Design review of the part built by this model. Coordinates are the model's own, in mm. A direction names the side the tool comes from. Round coordinates to 2 decimals unless told otherwise and drop trailing zeros. Loops run counter-clockwise (first coordinate to the right, second up) from the corner with the lowest first, then second, coordinate; pieces in that order, holes last. Notation, with made-up numbers: M 18,57 L 32,57 A29 ccw 32,96 Z; hole C -37.75,51 d7. An arc over 180 degrees is marked long. Use a Markdown table: item, result.
from build123d import *

# Parameters (mm, degrees)
SKETCH1_W           = 66.25
SKETCH1_H           = 78
SKETCH1_R           = 1.25
BOSS_EXTRUDE1_DEPTH = 3
SKETCH2_W           = 9.747388218
SKETCH2_H           = 78
SKETCH2_W_2         = 10.388237
BOSS_EXTRUDE2_DEPTH = 1.5
FILLET2_R           = 0.25
FILLET3_R           = 0.25
SKETCH3_R           = 2.3
SKETCH3_R_2         = 1.25
BOSS_EXTRUDE3_DEPTH = 4
SKETCH4_W           = 4.75
SKETCH4_H           = 3
BOSS_EXTRUDE4_DEPTH = 2
SKETCH5_W           = 5
SKETCH5_H           = 3
BOSS_EXTRUDE5_DEPTH = 30


with BuildPart() as part:
    # Sketch1 → Boss-Extrude1 (new body)
    with BuildSketch(Plane(origin=(0, 0, 0), x_dir=(1, 0, 0), z_dir=(0, 1, 0))):
        Rectangle(SKETCH1_W, SKETCH1_H)
        with Locations(Location((-21, 36, 0), (0, 0, 270))):
            Circle(SKETCH1_R, mode=Mode.SUBTRACT)
        with Locations(Location((21, 36, 0), (0, 0, 90))):
            Circle(SKETCH1_R, mode=Mode.SUBTRACT)
        with Locations(Location((21, -36, 0), (0, 0, 270))):
            Circle(SKETCH1_R, mode=Mode.SUBTRACT)
        with Locations(Location((-21, -36, 0), (0, 0, 90))):
            Circle(SKETCH1_R, mode=Mode.SUBTRACT)
    extrude(amount=BOSS_EXTRUDE1_DEPTH)

    # Sketch2 → Boss-Extrude2 (add)
    with BuildSketch(Plane.XZ):
        with Locations((-30.251305891, 0)):
            Rectangle(SKETCH2_W, SKETCH2_H)
        with Locations((29.9308815, 0)):
            Rectangle(SKETCH2_W_2, SKETCH2_H)
    extrude(amount=-BOSS_EXTRUDE2_DEPTH)

    # Fillet2
    fillet2_edges = [part.edges().sort_by_distance(p)[0] for p in [
        (-35.125, 0.75, 39),
        (-35.125, 0, 0),
        (-35.125, 1.5, 0),
        (-35.125, 0.75, -39),
    ]]
    fillet(fillet2_edges, radius=FILLET2_R)

    # Fillet3
    fillet3_edges = [part.edges().sort_by_distance(p)[0] for p in [
        (35.125, 0.75, -39),
        (35.125, 0, 0),
        (35.125, 1.5, 0),
        (35.125, 0.75, 39),
    ]]
    fillet(fillet3_edges, radius=FILLET3_R)

    # Sketch3 → Boss-Extrude3 (add)
    # profile 1 of 4: a face of its own
    with BuildSketch(Plane(origin=(0, 3, 0), x_dir=(1, 0, 0), z_dir=(0, 1, 0))):
        with Locations(Location((-21, 36, 0), (0, 0, 270))):
            Circle(SKETCH3_R)
        with Locations(Location((-21, 36, 0), (0, 0, 270))):
            Circle(SKETCH3_R_2, mode=Mode.SUBTRACT)
    # profile 2 of 4: a face of its own
    with BuildSketch(Plane(origin=(0, 3, 0), x_dir=(1, 0, 0), z_dir=(0, 1, 0))):
        with Locations(Location((21, 36, 0), (0, 0, 90))):
            Circle(SKETCH3_R)
        with Locations(Location((21, 36, 0), (0, 0, 90))):
            Circle(SKETCH3_R_2, mode=Mode.SUBTRACT)
    # profile 3 of 4: a face of its own
    with BuildSketch(Plane(origin=(0, 3, 0), x_dir=(1, 0, 0), z_dir=(0, 1, 0))):
        with Locations(Location((21, -36, 0), (0, 0, 270))):
            Circle(SKETCH3_R)
        with Locations(Location((21, -36, 0), (0, 0, 270))):
            Circle(SKETCH3_R_2, mode=Mode.SUBTRACT)
    # profile 4 of 4: a face of its own
    with BuildSketch(Plane(origin=(0, 3, 0), x_dir=(1, 0, 0), z_dir=(0, 1, 0))):
        with Locations(Location((-21, -36, 0), (0, 0, 90))):
            Circle(SKETCH3_R)
        with Locations(Location((-21, -36, 0), (0, 0, 90))):
            Circle(SKETCH3_R_2, mode=Mode.SUBTRACT)
    extrude(amount=BOSS_EXTRUDE3_DEPTH)

    # Sketch4 → Boss-Extrude4 (add)
    with BuildSketch(Plane.XY.offset(39)):
        with Locations((-20.925, 1.5)):
            Rectangle(SKETCH4_W, SKETCH4_H)
        with Locations((20.925, 1.5)):
            Rectangle(SKETCH4_W, SKETCH4_H)
    extrude(amount=BOSS_EXTRUDE4_DEPTH)

    # Sketch5 → Boss-Extrude5 (add)
    with BuildSketch(Plane(origin=(0, 0, -39), x_dir=(-1, 0, 0), z_dir=(0, 0, -1))):
        with Locations((-27.625, 1.5)):
            Rectangle(SKETCH5_W, SKETCH5_H)
        with Locations((27.625, 1.5)):
            Rectangle(SKETCH5_W, SKETCH5_H)
    extrude(amount=BOSS_EXTRUDE5_DEPTH)


solid = part.part
1. Machinability: for faces 4 (the face through (18.55, 1, 40)), 5 (the face through (30.125, 1, -54)), 6 (the face through (19.6, 4.972, 34.175)), 7 (the face through (-30.125, 1, -54)), which of the approach directions +Z, -Z, +X, -X, +Y, -Y give a long, thin tool a straight path to every point of the face, cutting with its end or side? Answer none if there is none.
Check values:
| item | result |
|---|---|
| face 4 | +Z, +Y, -Y |
| face 5 | -Z, +X, +Y, -Y |
| face 6 | +Y |
| face 7 | -Z, -X, +Y, -Y |
2. Wall thickness on line 1 along X through (y, z) = (6.75, -36); line 2 along X through (y, z) = (2, 36) (3 decimals); line 3 along X through (y, z) = (1.75, -62.5) (3 decimals): over which ranges is each line inside the solid? List them lowest first. Write a range as from..to.
Check values:
| item | result |
|---|---|
| line 1 | x = -23.3..-22.25, -19.75..-18.7, 18.7..19.75, 22.25..23.3 |
| line 2 | x = -33.125..-22.25, -19.75..19.75, 22.25..33.125 |
| line 3 | x = -30.125..-25.125, 25.125..30.125 |
3. Take a section at A-A on y = 5.75. Give the boundary of the cut face in (x, z).
Check values:
| item | result |
|---|---|
| outline | C -21,-36 d4.6; C -21,36 d4.6; C 21,-36 d4.6; C 21,36 d4.6; hole C -21,-36 d2.5; hole C -21,36 d2.5; hole C 21,-36 d2.5; hole C 21,36 d2.5 |
4. Take a section at B-B on z = -42. Give the boundary of the cut face in (x, y) (3 decimals).
Check values:
| item | result |
|---|---|
| outline | M -30.125,0 L -25.125,0 L -25.125,3 L -30.125,3 Z; M 25.125,0 L 30.125,0 L 30.125,3 L 25.125,3 Z |
5. Take a section at D-D on z = 36. Give the boundary of the cut face in (x, y) (3 decimals), and give its area (3 significant figures).
Check values:
| item | result |
|---|---|
| outline | M -35.125,0.25 A0.25 ccw -34.875,0 L -22.25,0 L -22.25,7 L -23.3,7 L -23.3,3 L -33.125,3 L -33.125,1.5 L -34.875,1.5 A0.25 ccw -35.125,1.25 Z; M -19.75,0 L 19.75,0 L 19.75,7 L 18.7,7 L 18.7,3 L -18.7,3 L -18.7,7 L -19.75,7 Z; M 22.25,0 L 34.875,0 A0.25 ccw 35.125,0.25 L 35.125,1.25 A0.25 ccw 34.875,1.5 L 33.125,1.5 L 33.125,3 L 23.3,3 L 23.3,7 L 22.25,7 Z |
| area | 206 mm² |
6. Insertion check: pin 1 (3.5 mm diameter, centred on y = 1, z = -52.5, fed in from -X) (3 decimals); pin 2 (1.4 mm diameter, centred on x = -34.5, z = 7.5, fed in from +Y); pin 3 (2.5 mm diameter, centred on y = 2, z = -46.5, fed in from +X) (3 decimals); pin 4 (3 mm diameter, centred on x = -12, z = 18.5, fed in from -Y). Each pin has a flat end and moves straight along its axis. Give the tip position at first contact, or say it passes through.
Check values:
| item | result |
|---|---|
| pin 1 | stops at x = -30.125 |
| pin 2 | stops at y = 1.5 |
| pin 3 | stops at x = 30.125 |
| pin 4 | stops at y = 0 |
7. The part is to be moulded in two halves that separate along X. For faces 1 (the face through (-19.6, 4.972, 37.825)), 2 (the face through (-23.3, 1, 40)), 3 (the face through (-29, 1, 39)), say which applies: pulls with the +X half, pulls with the -X half, needs draft (parallel to the pull), parting line crosses it, or undercut.
Check values:
| item | result |
|---|---|
| face 1 | undercut |
| face 2 | pulls with the -X half |
| face 3 | needs draft |
8. Take a section at C-C on x = -21. Give the boundary of the cut face in (y, z), and give its area (3 significant figures).
Check values:
| item | result |
|---|---|
| outline | M 0,-39 L 3,-39 L 3,-38.3 L 7,-38.3 L 7,-37.25 L 0,-37.25 Z; M 0,-34.75 L 7,-34.75 L 7,-33.7 L 3,-33.7 L 3,33.7 L 7,33.7 L 7,34.75 L 0,34.75 Z; M 0,37.25 L 7,37.25 L 7,38.3 L 3,38.3 L 3,41 L 0,41 Z |
| area | 242 mm² |
